Design review of the part built by this model. Coordinates are the model's own, in mm. Give positions to 0.01 mm unless a question says otherwise; leave off trailing zeros. Loops run counter-clockwise (first coordinate to the right, second up) from the corner with the lowest first, then second, coordinate; pieces in that order, holes last. Notation, with made-up numbers: (30, 64) -> (35, 64) arc R22 ccw to (35, 72) -> close; hole circle Ø3 at (42, 57). An arc over 180 degrees is marked (long way). Answer as CSV lines item,"result".
from build123d import *

# Parameters (mm, degrees)
F0_R     = 22.5
F1_DEPTH = 13
F3_D     = 10
F5_DEPTH = 25
F6_R     = 2


with BuildPart() as f1:
    # F0 (on Front) → F1 (new body)
    with BuildSketch(Plane.XZ):
        Circle(F0_R)
    extrude(amount=F1_DEPTH)

    # F3 (through all)
    with Locations(Plane.XZ.offset(13)):
        with Locations((0, 0)):
            Hole(F3_D / 2)

    # F4 (on face) → F5 (cut)
    with BuildSketch(Plane.XZ.offset(13)):
        with BuildLine():
            Line((-18.6533453825, -12.5818403281), (-12.8500823746, -8.6674900038))
            ThreePointArc((-12.8500823746, -8.6674900038), (-16.9085134828, -4.9854002249), (-22.2102103191, -3.5995218548))
            ThreePointArc((-22.2102103191, -3.5995218548), (-20.9195615975, -8.2838362229), (-18.6533453825, -12.5818403281))
        make_face()
        with BuildLine():
            ThreePointArc((-11.6575097746, -19.2445437944), (-11.0790420161, -17.2071413146), (-10.884014459, -15.0982083937))
            ThreePointArc((-10.884014459, -15.0982083937), (-11.3865097654, -11.7359337894), (-12.8500823746, -8.6674900038))
            Line((-12.8500823746, -8.6674900038), (-18.6533453825, -12.5818403281))
            ThreePointArc((-18.6533453825, -12.5818403281), (-15.5172449055, -16.29310009), (-11.6575097746, -19.2445437944))
        make_face()
        with BuildLine():
            ThreePointArc((19.2445437944, -11.6575097746), (8.6674900038, -12.8500823746), (3.5995218548, -22.2102103191))
            ThreePointArc((3.5995218548, -22.2102103191), (12.5818403281, -18.6533453825), (19.2445437944, -11.6575097746))
        make_face()
        with BuildLine():
            ThreePointArc((22.2102103191, 3.5995218548), (18.6533453825, 12.5818403281), (11.6575097746, 19.2445437944))
            ThreePointArc((11.6575097746, 19.2445437944), (12.8500823746, 8.6674900038), (22.2102103191, 3.5995218548))
        make_face()
        with BuildLine():
            ThreePointArc((-3.5995218548, 22.2102103191), (-12.5818403281, 18.6533453825), (-19.2445437944, 11.6575097746))
            ThreePointArc((-19.2445437944, 11.6575097746), (-8.6674900038, 12.8500823746), (-3.5995218548, 22.2102103191))
        make_face()
    extrude(amount=-F5_DEPTH, mode=Mode.SUBTRACT)

    # F6
    f6_edges = [f1.edges().sort_by_distance(p)[0] for p in [
        (8.66749, -13, -12.850082),
        (22.086612, -13, -4.293202),
        (12.850082, -13, 8.66749),
        (4.293202, -13, 22.086612),
        (-8.66749, -13, 12.850082),
        (-22.086612, -13, 4.293202),
        (-12.850082, -13, -8.66749),
        (-4.293202, -13, -22.086612),
        (-5, -13, 0),
    ]]
    fillet(f6_edges, radius=F6_R)


solid = f1.part
Q1. We need section C-C, the plane y = -4.5. State the section outline as (x, z) points, and give its area (3 significant figures).
Filled sheet:
outline,"(-22.21, -3.6) arc R11.5 cw to (-11.66, -19.24) arc R22.5 ccw to (3.6, -22.21) arc R11.5 cw to (19.24, -11.66) arc R22.5 ccw to (22.21, 3.6) arc R11.5 cw to (11.66, 19.24) arc R22.5 ccw to (-3.6, 22.21) arc R11.5 cw to (-19.24, 11.66) arc R22.5 ccw to start; hole circle Ø10 at (0, 0)"
area,"1,150 mm^2"
Q2. We need section B-B, the plane x = 0. State the section outline as (y, z) points.
Filled sheet:
outline,"(-13, -20.5) arc R2 ccw to (-11, -22.5) -> (0, -22.5) -> (0, -5) -> (-11, -5) arc R2 ccw to (-13, -7) -> close; (-13, 7) arc R2 ccw to (-11, 5) -> (0, 5) -> (0, 22.5) -> (-11, 22.5) arc R2 ccw to (-13, 20.5) -> close"
Q3. To check wall thickness, follow probe 1 along Z at (x, y) = (0, -3); probe 2 along Y at (x, z) = (-5.5, -3); probe 3 along X at (y, z) = (-11.25, 1.5). State the ranges of each line that lie inside material, in increasing order. Write a range as from..to.
Filled sheet:
probe 1,"z = -22.5..-5, 5..22.5"
probe 2,"y = -12.86..0"
probe 3,"x = -22.43..-4.79, 4.79..22.43"
Q4. We need section D-D, the plane y = -11.75. State the section outline as (x, z) points, and give its area (3 significant figures).
Filled sheet:
outline,"(-22.09, -3.46) arc R11.65 cw to (-11.48, -19.18) arc R22.35 ccw to (3.46, -22.09) arc R11.65 cw to (19.18, -11.48) arc R22.35 ccw to (22.09, 3.46) arc R11.65 cw to (11.48, 19.18) arc R22.35 ccw to (-3.46, 22.09) arc R11.65 cw to (-19.18, 11.48) arc R22.35 ccw to start; hole circle Ø10.29 at (0, 0)"
area,"1,120 mm^2"
Q5. We need section A-A, the plane z = 0. State the section outline as (x, y) points.
Filled sheet:
outline,"(-22.5, -11) arc R2 ccw to (-20.5, -13) -> (-7, -13) arc R2 ccw to (-5, -11) -> (-5, 0) -> (-22.5, 0) -> close; (5, -11) arc R2 ccw to (7, -13) -> (20.5, -13) arc R2 ccw to (22.5, -11) -> (22.5, 0) -> (5, 0) -> close"
Q6. The part is to be moulded in two halves that separate along X. For faces 1 (the cylindrical face through (-22.065, -5.423, 4.402)), 2 (the flat face through (9, -13, 0)), 3 (the cylindrical face through (8.8, -5.58, -12.76)), 4 (the cylindrical face through (-4.402, -5.423, -22.065)), say which applies: pulls with the +X half, pulls with the -X half, needs draft (parallel to the pull), parting line crosses it, or undercut.
Filled sheet:
face 1,"pulls with the -X half"
face 2,"needs draft"
face 3,"undercut"
face 4,"parting line crosses it"
Q7. Clearance check with flat-ended pins moving along their axes: pin 1 Ø4 at (y, z) = (-5, 17) entering from -X; pin 2 Ø6 at (y, z) = (-5.5, -7) entering from +X; pin 3 Ø9 at (x, z) = (0, 0) entering from +Y; pin 4 Ø3 at (x, y) = (-7, -10) entering from +Z. State where each tip first meets the part, or that it passes through.
Filled sheet:
pin 1,"stops at x = -6.28"
pin 2,"stops at x = 22.14"
pin 3,"passes through"
pin 4,"stops at z = 16.05"
